from build123d import *

# Parameters (mm, degrees)
SKETCH1_W           = 107.95
SKETCH1_H           = 127.508
SKETCH1_R           = 25.4
SKETCH1_R_2         = 3.175
BOSS_EXTRUDE1_DEPTH = 6.35


with BuildPart() as part:
    # Sketch1 → Boss-Extrude1 (new body)
    with BuildSketch(Plane.XY):
        with Locations((0, 21.971)):
            Rectangle(SKETCH1_W, SKETCH1_H)
        Circle(SKETCH1_R, mode=Mode.SUBTRACT)
        with Locations((-44.45, 76.2)):
            Circle(SKETCH1_R_2, mode=Mode.SUBTRACT)
        with Locations((44.45, 76.2)):
            Circle(SKETCH1_R_2, mode=Mode.SUBTRACT)
        with Locations((-44.45, 12.7)):
            Circle(SKETCH1_R_2, mode=Mode.SUBTRACT)
        with Locations((-44.45, -12.7)):
            Circle(SKETCH1_R_2, mode=Mode.SUBTRACT)
        with Locations((44.45, -12.7)):
            Circle(SKETCH1_R_2, mode=Mode.SUBTRACT)
        with Locations((44.45, 12.7)):
            Circle(SKETCH1_R_2, mode=Mode.SUBTRACT)
    extrude(amount=BOSS_EXTRUDE1_DEPTH)


solid = part.part
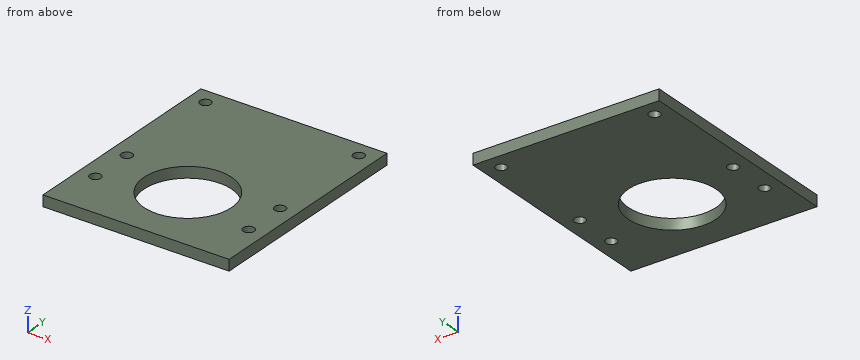
CAD build for the part. Positions are in the model's coordinates, mm. Coordinates: 2 decimals unless noted, no trailing zeros. Write each loop counter-clockwise with the first axis right and the second up, starting at its lowest first coordinate (ties: lowest second). Pieces come first, ordered by that corner, then holes. Notation, with made-up numbers: M -16.5,64.25 L -8.5,64.25 A23 ccw -8.5,86.25 Z; hole C 81.5,-35.75 d4. An arc over 180 degrees is marked long. Answer as a JSON object with one key per item and string values. Group by question number.
1) Pin check, flat tip, straight feed: pin 1 Ø8.5 at (x, y) = (-44.45, 12.7) entering from -Z. Stop position of the tip, or through.
2) Saw through at C-C (y = 12.7). Write the cut outline in (x, z) (3 decimals), plus the area to 3 significant figures.
3) Saw through at D-D (z = 1). Write the cut outline in (x, y) (3 decimals).
4) Wall check: line 1 (Y direction, x = 44.45, z = 3.25) (3 decimals); line 2 (Y direction, x = 43.5, z = 6.25) (3 decimals); line 3 (X direction, y = 1, z = 4.5) (3 decimals). Give the ranges that are in metal, low to high. Write a range as from..to.
5) Saw through at A-A (x = 0). Write the cut outline in (y, z) (3 decimals), plus the area to 3 significant figures.
6) Saw through at B-B (x = -44.45). Write the cut outline in (y, z) (3 decimals).
Values follow:
{
 "1": {"pin 1": "stops at z = 0"},
 "2": {"outline": "M -53.975,0 L -47.625,0 L -47.625,6.35 L -53.975,6.35 Z; M -41.275,0 L -21.997,0 L -21.997,6.35 L -41.275,6.35 Z; M 21.997,0 L 41.275,0 L 41.275,6.35 L 21.997,6.35 Z; M 47.625,0 L 53.975,0 L 53.975,6.35 L 47.625,6.35 Z", "area": "325 mm2"},
 "3": {"outline": "M -53.975,-41.783 L 53.975,-41.783 L 53.975,85.725 L -53.975,85.725 Z; hole C -44.45,-12.7 d6.35; hole C -44.45,12.7 d6.35; hole C -44.45,76.2 d6.35; hole C 0,0 d50.8; hole C 44.45,-12.7 d6.35; hole C 44.45,12.7 d6.35; hole C 44.45,76.2 d6.35"},
 "4": {"line 1": "y = -41.783..-15.875, -9.525..9.525, 15.875..73.025, 79.375..85.725", "line 2": "y = -41.783..-15.73, -9.67..9.67, 15.73..73.17, 79.23..85.725", "line 3": "x = -53.975..-25.38, 25.38..53.975"},
 "5": {"outline": "M -41.783,0 L -25.4,0 L -25.4,6.35 L -41.783,6.35 Z; M 25.4,0 L 85.725,0 L 85.725,6.35 L 25.4,6.35 Z", "area": "487 mm2"},
 "6": {"outline": "M -41.783,0 L -15.875,0 L -15.875,6.35 L -41.783,6.35 Z; M -9.525,0 L 9.525,0 L 9.525,6.35 L -9.525,6.35 Z; M 15.875,0 L 73.025,0 L 73.025,6.35 L 15.875,6.35 Z; M 79.375,0 L 85.725,0 L 85.725,6.35 L 79.375,6.35 Z"}
}
